```python
from build123d import *

# Parameters (mm, degrees)
SKETCH1_W                                       = 82.55
SKETCH1_H                                       = 111.125
BOSS_EXTRUDE1_DEPTH                             = 19.05
SKETCH14_W                                      = 76.2
SKETCH14_H                                      = 101.6
CUT_EXTRUDE3_DEPTH                              = 15.875
CUT_EXTRUDE4_REACH                              = 113.125
SKETCH11_R                                      = 7.1501
SKETCH17_W                                      = 76.2
SKETCH17_H                                      = 6.35
BOSS_EXTRUDE4_DEPTH                             = 10.3251
SKETCH18_R                                      = 5.953125
CUT_EXTRUDE5_DEPTH                              = 6.35
CUT_EXTRUDE5_TAPER                              = 5
CUT_EXTRUDE7_REACH                              = 113.125
FILLET6_R                                       = 1.5875
SKETCH19_R                                      = 2.8575
BOSS_EXTRUDE8_DEPTH                             = 3.175
CBORE_FOR_4_PAN_HEAD_MACHINE_SCREW3_D           = 3.2639
CBORE_FOR_4_PAN_HEAD_MACHINE_SCREW3_CBORE_D     = 6.35
CBORE_FOR_4_PAN_HEAD_MACHINE_SCREW3_CBORE_DEPTH = 2.032
F_4_40_TAPPED_HOLE1_D                           = 2.2606
F_4_40_TAPPED_HOLE1_DEPTH                       = 4.7752
F_4_40_TAPPED_HOLE1_TIP                         = 0.679152758
SKETCH39_W                                      = 17.4625
SKETCH39_H                                      = 14.2875
CUT_EXTRUDE8_DEPTH                              = 1.5875
FILLET7_R                                       = 0.79375
FILLET8_R                                       = 0.1984375
FILLET9_R                                       = 0.396875
SKETCH40_W                                      = 10.03389441
SKETCH40_H                                      = 4.365625
BOSS_EXTRUDE9_DEPTH                             = 1.5875
FILLET10_R                                      = 1.5875
SKETCH41_W                                      = 76.2
SKETCH41_H                                      = 6.35
CUT_EXTRUDE9_DEPTH                              = 1.5875


with BuildPart() as part:
    # Sketch1 → Boss-Extrude1 (new body)
    with BuildSketch(Plane(origin=(0, 0, 0), x_dir=(1, 0, 0), z_dir=(0, 1, 0))):
        Rectangle(SKETCH1_W, SKETCH1_H)
    extrude(amount=BOSS_EXTRUDE1_DEPTH)

    # Sketch14 → Cut-Extrude3 (cut)
    with BuildSketch(Plane(origin=(0, 19.05, 0), x_dir=(-1, 0, 0), z_dir=(0, 1, 0))):
        with Locations((0, -1.5875)):
            Rectangle(SKETCH14_W, SKETCH14_H)
    extrude(amount=-CUT_EXTRUDE3_DEPTH, mode=Mode.SUBTRACT)

    # Sketch11 → Cut-Extrude4 (cut, up to next)
    with BuildSketch(Plane.XY.offset(55.5625), mode=Mode.PRIVATE) as cut_extrude4_sk1:
        with Locations((-28.575, 13.5001)):
            Circle(SKETCH11_R)
    cut_extrude4_tool1 = extrude(cut_extrude4_sk1.sketch, amount=-CUT_EXTRUDE4_REACH, mode=Mode.PRIVATE) & part.part
    add(cut_extrude4_tool1.solids().sort_by_distance((-28.575, 13.5001, 55.5625))[0], mode=Mode.SUBTRACT)
    # Sketch11 → Cut-Extrude4 (cut, up to next)
    with BuildSketch(Plane.XY.offset(55.5625), mode=Mode.PRIVATE) as cut_extrude4_sk2:
        with Locations((-9.525, 13.5001)):
            Circle(SKETCH11_R)
    cut_extrude4_tool2 = extrude(cut_extrude4_sk2.sketch, amount=-CUT_EXTRUDE4_REACH, mode=Mode.PRIVATE) & part.part
    add(cut_extrude4_tool2.solids().sort_by_distance((-9.525, 13.5001, 55.5625))[0], mode=Mode.SUBTRACT)
    # Sketch11 → Cut-Extrude4 (cut, up to next)
    with BuildSketch(Plane.XY.offset(55.5625), mode=Mode.PRIVATE) as cut_extrude4_sk3:
        with Locations((9.525, 13.5001)):
            Circle(SKETCH11_R)
    cut_extrude4_tool3 = extrude(cut_extrude4_sk3.sketch, amount=-CUT_EXTRUDE4_REACH, mode=Mode.PRIVATE) & part.part
    add(cut_extrude4_tool3.solids().sort_by_distance((9.525, 13.5001, 55.5625))[0], mode=Mode.SUBTRACT)
    # Sketch11 → Cut-Extrude4 (cut, up to next)
    with BuildSketch(Plane.XY.offset(55.5625), mode=Mode.PRIVATE) as cut_extrude4_sk4:
        with Locations((28.575, 13.5001)):
            Circle(SKETCH11_R)
    cut_extrude4_tool4 = extrude(cut_extrude4_sk4.sketch, amount=-CUT_EXTRUDE4_REACH, mode=Mode.PRIVATE) & part.part
    add(cut_extrude4_tool4.solids().sort_by_distance((28.575, 13.5001, 55.5625))[0], mode=Mode.SUBTRACT)

    # Sketch17 → Boss-Extrude4 (add)
    with BuildSketch(Plane(origin=(0, 3.175, 0), x_dir=(-1, 0, 0), z_dir=(0, 1, 0))):
        with Locations((0, 15.08125)):
            Rectangle(SKETCH17_W, SKETCH17_H)
        with BuildLine():
            Line((32.146875, -49.2125), (32.146875, -52.3875))
            Line((32.146875, -52.3875), (38.1, -52.3875))
            Line((38.1, -52.3875), (38.1, -46.434375))
            Line((38.1, -46.434375), (34.925, -46.434375))
            ThreePointArc((34.925, -46.434375), (32.960568974, -47.248068974), (32.146875, -49.2125))
        make_face()
        with BuildLine():
            Line((-32.146875, -49.2125), (-32.146875, -52.3875))
            Line((-32.146875, -52.3875), (-38.1, -52.3875))
            Line((-38.1, -52.3875), (-38.1, -46.434375))
            Line((-38.1, -46.434375), (-34.925, -46.434375))
            ThreePointArc((-34.925, -46.434375), (-32.960568974, -47.248068974), (-32.146875, -49.2125))
        make_face()
    extrude(amount=BOSS_EXTRUDE4_DEPTH)

    # Sketch18 → Cut-Extrude5 (cut)
    with BuildSketch(Plane.XY.offset(18.25625)):
        with Locations((-28.575, 13.5001)):
            Circle(SKETCH18_R)
        with Locations((-9.525, 13.5001)):
            Circle(SKETCH18_R)
        with Locations((9.525, 13.5001)):
            Circle(SKETCH18_R)
        with Locations((28.575, 13.5001)):
            Circle(SKETCH18_R)
    extrude(amount=-CUT_EXTRUDE5_DEPTH, taper=CUT_EXTRUDE5_TAPER, mode=Mode.SUBTRACT)

    # Sketch21 → Cut-Extrude7 (cut, up to next)
    with BuildSketch(Plane(origin=(0, 0, -55.5625), x_dir=(-1, 0, 0), z_dir=(0, 0, -1)), mode=Mode.PRIVATE) as cut_extrude7_sk1:
        Polygon((-3.683, 7.9375), (-3.683, 9.525), (-4.1671875, 9.525), (-4.1671875, 12.1046875), (4.1671875, 12.1046875), (4.1671875, 9.525), (3.683, 9.525), (3.683, 7.9375), align=None)
    cut_extrude7_tool1 = extrude(cut_extrude7_sk1.sketch, amount=-CUT_EXTRUDE7_REACH, mode=Mode.PRIVATE) & part.part
    add(cut_extrude7_tool1.solids().sort_by_distance((0, 10.08083, -55.5625))[0], mode=Mode.SUBTRACT)

    # Fillet6
    fillet6_edges = [part.edges().sort_by_distance(p)[0] for p in [
        (0, 0, 55.5625),
        (-41.275, 0, 0),
        (0, 0, -55.5625),
        (41.275, 0, 0),
        (41.275, 9.525, 55.5625),
        (-41.275, 9.525, 55.5625),
        (-41.275, 9.525, -55.5625),
        (41.275, 9.525, -55.5625),
    ]]
    fillet(fillet6_edges, radius=FILLET6_R)

    # Sketch19 → Boss-Extrude8 (add)
    with BuildSketch(Plane(origin=(0, 3.175, 0), x_dir=(-1, 0, 0), z_dir=(0, 1, 0))):
        with Locations((8.255, -48.5775)):
            Circle(SKETCH19_R)
        with Locations((-8.255, -48.5775)):
            Circle(SKETCH19_R)
        with Locations((17.78, -18.0975)):
            Circle(SKETCH19_R)
        with Locations((-17.78, -18.0975)):
            Circle(SKETCH19_R)
    extrude(amount=BOSS_EXTRUDE8_DEPTH)

    # CBORE for #4 Pan Head Machine Screw3 (through all)
    with Locations(Plane.XZ):
        with Locations((-19.05, 15.08125), (19.05, 15.08125), (-34.925, -49.2125), (34.925, -49.2125)):
            CounterBoreHole(CBORE_FOR_4_PAN_HEAD_MACHINE_SCREW3_D / 2, CBORE_FOR_4_PAN_HEAD_MACHINE_SCREW3_CBORE_D / 2, CBORE_FOR_4_PAN_HEAD_MACHINE_SCREW3_CBORE_DEPTH)

    # #4-40 Tapped Hole1
    with Locations(Plane(origin=(-31.823802028, 6.35, 11.997353854), x_dir=(-1, 0, 0), z_dir=(0, 1, 0))):
        with Locations((-23.568802028, -60.574853854), (-14.043802028, -30.094853854), (-49.603802028, -30.094853854), (-40.078802028, -60.574853854)):
            Hole(F_4_40_TAPPED_HOLE1_D / 2, depth=F_4_40_TAPPED_HOLE1_DEPTH)
            with Locations((0, 0, -(F_4_40_TAPPED_HOLE1_DEPTH + F_4_40_TAPPED_HOLE1_TIP / 2))):  # 118° drill point
                Cone(0, F_4_40_TAPPED_HOLE1_D / 2, F_4_40_TAPPED_HOLE1_TIP, mode=Mode.SUBTRACT)

    # Sketch39 → Cut-Extrude8 (cut)
    with BuildSketch(Plane(origin=(0, 0, -55.5625), x_dir=(-1, 0, 0), z_dir=(0, 0, -1))):
        with Locations((0, 10.02109375)):
            Rectangle(SKETCH39_W, SKETCH39_H)
    extrude(amount=-CUT_EXTRUDE8_DEPTH, mode=Mode.SUBTRACT)

    # Fillet7
    fillet7_edges = [part.edges().sort_by_distance(p)[0] for p in [
        (-8.73125, 17.16484375, -54.76875),
        (-8.73125, 2.87734375, -54.76875),
        (8.73125, 2.87734375, -54.76875),
        (8.73125, 17.16484375, -54.76875),
    ]]
    fillet(fillet7_edges, radius=FILLET7_R)

    # Fillet8
    fillet8_edges = [part.edges().sort_by_distance(p)[0] for p in [
        (3.683, 9.525, -53.18125),
        (4.1671875, 9.525, -53.18125),
        (-4.1671875, 9.525, -53.18125),
        (-3.683, 9.525, -53.18125),
    ]]
    fillet(fillet8_edges, radius=FILLET8_R)

    # Fillet9
    fillet9_edges = [part.edges().sort_by_distance(p)[0] for p in [
        (-3.683, 7.9375, -53.18125),
        (3.683, 7.9375, -53.18125),
        (4.1671875, 12.1046875, -53.18125),
        (-4.1671875, 12.1046875, -53.18125),
    ]]
    fillet(fillet9_edges, radius=FILLET9_R)

    # Sketch40 → Boss-Extrude9 (add)
    with BuildSketch(Plane(origin=(0, 19.05, 0), x_dir=(1, 0, 0), z_dir=(0, 1, 0))):
        Polygon((-33.083052795, -49.2125), (-33.083052795, -53.578125), (-39.290625, -53.578125), (-39.290625, 53.578125), (39.290625, 53.578125), (39.290625, -53.578125), (33.083052795, -53.578125), (33.083052795, -49.2125), (38.1, -49.2125), (38.1, 52.3875), (-38.1, 52.3875), (-38.1, -49.2125), align=None)
        with Locations((-19.05, -51.3953125)):
            Rectangle(SKETCH40_W, SKETCH40_H)
        with Locations((0, -51.3953125)):
            Rectangle(SKETCH40_W, SKETCH40_H)
        with Locations((19.05, -51.3953125)):
            Rectangle(SKETCH40_W, SKETCH40_H)
    extrude(amount=BOSS_EXTRUDE9_DEPTH)

    # Fillet10
    fillet10_edges = [part.edges().sort_by_distance(p)[0] for p in [
        (-39.290625, 19.84375, -53.578125),
        (-39.290625, 19.84375, 53.578125),
        (39.290625, 19.84375, 53.578125),
        (39.290625, 19.84375, -53.578125),
    ]]
    fillet(fillet10_edges, radius=FILLET10_R)

    # Sketch41 → Cut-Extrude9 (cut)
    with BuildSketch(Plane(origin=(0, 13.5001, 0), x_dir=(1, 0, 0), z_dir=(0, 1, 0))):
        with Locations((0, -15.08125)):
            Rectangle(SKETCH41_W, SKETCH41_H)
    extrude(amount=-CUT_EXTRUDE9_DEPTH, mode=Mode.SUBTRACT)


solid = part.part
```
Check sheet for the modelled part. Datum: model origin and axes. Units: mm. A direction names the side the tool comes from. Round coordinates to 2 decimals unless told otherwise and drop trailing zeros. Write item = value, one per line. Start each with the question number.
1. Tool access check on faces 3 (the conical face through (28.47, 7.83, 15.04)), 4 (the cylindrical face through (18.3, 3.9, -19.1)), 5 (the flat face through (33, 2.032, -48)). Record the directions out of +Z, -Z, +X, -X, +Y, -Y that give a thin tool (end or side, any length) a straight path to the whole face; none if there is none.
2. Gauge pin test, flat ends, axial feed: pin 1 (10 mm diameter, centred on x = 8, z = 4.5, fed in from +Y) (3 decimals); pin 2 (1.8 mm diameter, centred on x = -8.25, z = -48.58, fed in from -Y); pin 3 (6 mm diameter, centred on x = -9, y = 14.5, fed in from +Z); pin 4 (1.9 mm diameter, centred on x = -18, z = 14.5, fed in from +Y). Record the tip position at first contact, or that the pin passes through.
3. Scan lines: line 1 (Z direction, x = -3, y = 5.25) (1 decimal); line 2 (Z direction, x = -15.5, y = 6.5); line 3 (X direction, y = 9.25, z = 22) (3 decimals). Record each from-to range of solid material in increasing order. Write a range as [from, to].
4. Release check for a two-part mould opening along X. For faces 1 (the conical face through (8.298, 1.014, -48.769)), 2 (the flat face through (19, 20.638, 51)) record: pulls with the +X half, pulls with the -X half, needs draft (parallel to the pull), parting line crosses it, or undercut.
Results found:
q1.face_3 = +Z, +Y
q1.face_4 = +Y
q1.face_5 = -Y
q2.pin_1 = 3.175
q2.pin_2 = 0
q2.pin_3 = -52.39
q2.pin_4 = 11.91
q3.line_1 = [-54, -52.4], [11.9, 18.3], [49.2, 55.6]
q3.line_2 = [-55.56, -52.39], [11.91, 18.26], [49.21, 55.56]
q3.line_3 = [-41.275, -38.1], [38.1, 41.275]
q4.face_1 = undercut
q4.face_2 = needs draft
